Check sheet for the modelled part. Datum: model origin and axes. Units: mm. A direction names the side the tool comes from. Give positions to 0.01 mm unless a question says otherwise; leave off trailing zeros. Order: outer loops, then holes, each group sorted by start corner. A loop starts at its lowest first (then second) coordinate and runs counter-clockwise, first axis right, second up. Notation, with made-up numbers: (12.25, 43) - (19.25, 43) arc R26 ccw to (19.25, 74) - close; hole circle Ø7 at (-13.5, 79). An arc over 180 degrees is marked (long way). Answer in a Markdown table with one row per item.
from build123d import *

# Parameters (mm, degrees)
FILLET1_R   = 0.2
HEX_2_DEPTH = 2.5


with BuildPart() as part:
    # BodySke → Base-Revolve (revolve)
    with BuildSketch(Plane.XY):
        Polygon((0, 0), (0, 3.75), (0.5, 4.25), (4, 4.25), (4, 2.5), (14.555, 2.5), (15, 2.055), (15, 0), align=None)
    revolve(axis=Axis((-31.75, 0, 0), (1, 0, 0)))

    # Fillet1
    fillet1_edges = [part.edges().sort_by_distance(p)[0] for p in [
        (4, -2.5, 0),
    ]]
    fillet(fillet1_edges, radius=FILLET1_R)

    # Sketch2 → Hex-PreBroach (revolve, cut)
    with BuildSketch(Plane.XY):
        Polygon((0, 2.042), (2.5, 2.042), (3.67894925, 0), (0, 0), align=None)
    revolve(axis=Axis((0, 0, 0), (1, 0, 0)), mode=Mode.SUBTRACT)

    # Sketch3 → Hex 2 (cut)
    with BuildSketch(Plane(origin=(0, 0, 0), x_dir=(0, 0.5, 0.866025404), z_dir=(-1, 0, 0))):
        Polygon((1.17894925, 2.042), (-1.17894925, 2.042), (-2.357898499, 0), (-1.17894925, -2.042), (1.17894925, -2.042), (2.357898499, 0), align=None)
    extrude(amount=-HEX_2_DEPTH, mode=Mode.SUBTRACT)


solid = part.part
(1) Thickness scan on L1, parallel to X at y = -1.75, z = 2; L2, parallel to Z at x = 1, y = 2; L3, parallel to X at y = 1, z = -2. Record the ranges inside material, lowest first.
Geometry says:
| item | result |
|---|---|
| L1 | 0 to 4 |
| L2 | -3.75 to -0.62, 0.62 to 3.75 |
| L3 | 2.5 to 14.82 |
(2) Cross-section at A-A, the plane x = 11.25. Record the cut outline in (y, z).
Geometry says:
| item | result |
|---|---|
| outline | circle Ø5 at (0, 0) |
(3) Access from +Z, -Z, +X, -X, +Y, -Y to the whole of each face (thin tool, end or side, straight path). Record for faces 5 (the flat face through (1.232, 1.777, -1.007)), 6 (the flat face through (15, 0, 0)), 7 (the cylindrical face through (9.45, -0.54, -2.44)).
Geometry says:
| item | result |
|---|---|
| face 5 | -X |
| face 6 | +Z, -Z, +X, +Y, -Y |
| face 7 | +X |
(4) Mould release check, pull along Z, two halves, no side actions. Record for faces 1 (the cylindrical face through (2.274, 2.285, 3.584)), 2 (the flat face through (4, 0, -3)), 3 (the flat face through (1.232, -1.777, 1.007)), 4 (the conical face through (3.49, -0.07, -0.32)): pulls with the +Z half, pulls with the -Z half, needs draft (parallel to the pull), parting line crosses it, or undercut.
Geometry says:
| item | result |
|---|---|
| face 1 | parting line crosses it |
| face 2 | needs draft |
| face 3 | undercut |
| face 4 | undercut |
(5) Cross-section at B-B, the plane x = 2.75. Record the cut outline in (y, z).
Geometry says:
| item | result |
|---|---|
| outline | circle Ø8.5 at (0, 0); hole circle Ø3.22 at (0, 0) |
(6) Gauge pin test, flat ends, axial feed: P1, Ø5, axis at x = 10, y = 1, coming from the -Z side; P2, Ø0.7, axis at x = 0.5, y = 0.5, coming from the -Z side; P3, Ø1, axis at x = 10.5, z = 2.5, coming from the +Y side. Record the tip position at first contact, or that the pin passes through.
Geometry says:
| item | result |
|---|---|
| P1 | z = -2.5 |
| P2 | z = -4.25 |
| P3 | y = 1.5 |
